The drawing under review shows one solid part. Ordinate dimensions are in mm from its lowest x, y, z. Coordinates: 2 decimals unless noted, no trailing zeros. Order: outer loops, then holes, each group sorted by start corner. A loop starts at its lowest first (then second) coordinate and runs counter-clockwise, first axis right, second up. Notation, with made-up numbers: (-19, -19) -> (4, -19) arc R31 cw to (4, 14) -> close; hole circle Ø5 at (67.5, -24). An arc over 180 degrees is marked (long way). Use one line per item in the form item = value.
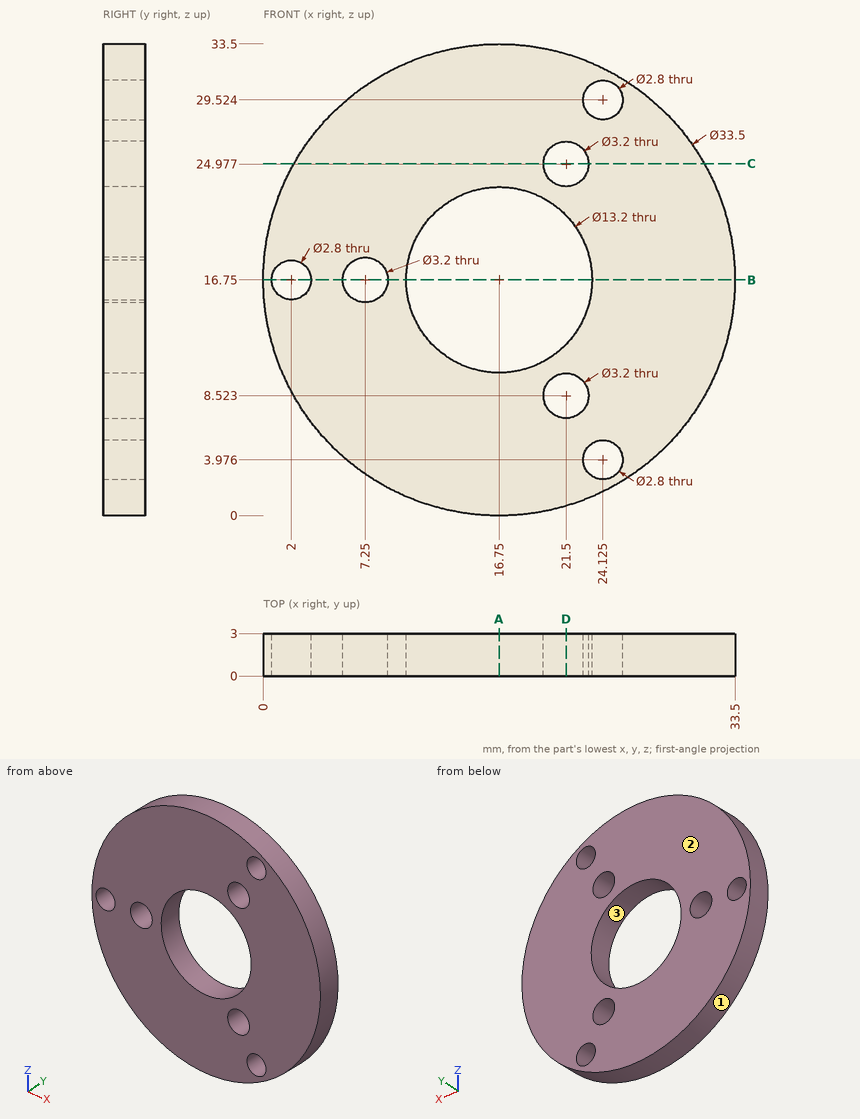
Item 1: Draft analysis for pull direction X (two halves, no side actions). For the marked faces 1, 2 and 3, state which applies: released by +X, released by -X, zero draft, split by the parting line, or undercut.
Results found:
face_1 = split by the parting line
face_2 = zero draft
face_3 = undercut
Item 2: We need section D-D (x = 21.5). Write out the cut boundary in (y, z).
Results found:
outline = (0, 0.69) -> (3, 0.69) -> (3, 6.92) -> (0, 6.92) -> close; (0, 10.12) -> (3, 10.12) -> (3, 12.17) -> (0, 12.17) -> close; (0, 21.33) -> (3, 21.33) -> (3, 23.38) -> (0, 23.38) -> close; (0, 26.58) -> (3, 26.58) -> (3, 32.81) -> (0, 32.81) -> close
Item 3: We need section B-B (z = 16.75). Write out the cut boundary in (x, y).
Results found:
outline = (0, 0) -> (0.6, 0) -> (0.6, 3) -> (0, 3) -> close; (3.4, 0) -> (5.65, 0) -> (5.65, 3) -> (3.4, 3) -> close; (8.85, 0) -> (10.15, 0) -> (10.15, 3) -> (8.85, 3) -> close; (23.35, 0) -> (33.5, 0) -> (33.5, 3) -> (23.35, 3) -> close
Item 4: We need section C-C (z = 25). Write out the cut boundary in (x, y).
Results found:
outline = (2.17, 0) -> (19.9, 0) -> (19.9, 3) -> (2.17, 3) -> close; (23.1, 0) -> (31.33, 0) -> (31.33, 3) -> (23.1, 3) -> close
Item 5: Clearance check with flat-ended pins moving along their axes: pin 1 (1.5 mm diameter, centred on x = 20, y = 1, fed in from +Z); pin 2 (1.5 mm diameter, centred on y = 2, z = 24.5, fed in from +X); pin 3 (1.7 mm diameter, centred on x = 24.12, z = 3.98, fed in from +Y); pin 4 (1 mm diameter, centred on x = 7.5, y = 0.5, fed in from +Z). State where each tip first meets the part, or that it passes through.
Results found:
pin_1 = 33.31
pin_2 = 31.97
pin_3 = through
pin_4 = 31.03
Item 6: To check wall thickness, follow L1, parallel to X at y = 1.6, z = 16.75; L2, parallel to X at y = 1.4, z = 22.5; L3, parallel to X at y = 1.2, z = 13 (1 decimal). State the ranges of each line that lie inside material, in increasing order. Write a range as from..to.
Results found:
L1 = 0..0.6, 3.4..5.65, 8.85..10.15, 23.35..33.5
L2 = 1.02..13.51, 19.99..32.48
L3 = 0.4..11.3, 22.2..33.1
Item 7: We need section A-A (x = 16.75). Write out the cut boundary in (y, z), plus the area to 3 significant figures.
Results found:
outline = (0, 0) -> (3, 0) -> (3, 10.15) -> (0, 10.15) -> close; (0, 23.35) -> (3, 23.35) -> (3, 33.5) -> (0, 33.5) -> close
area = 60.9 mm²
